Can you work these out from the drawing? Everything is in mm from the part's minimum corner. A direction names the side the tool comes from. Coordinates: 2 decimals unless noted, no trailing zeros. Loops run counter-clockwise (first coordinate to the right, second up) from the corner with the lowest first, then second, coordinate; pieces in that order, holes last.
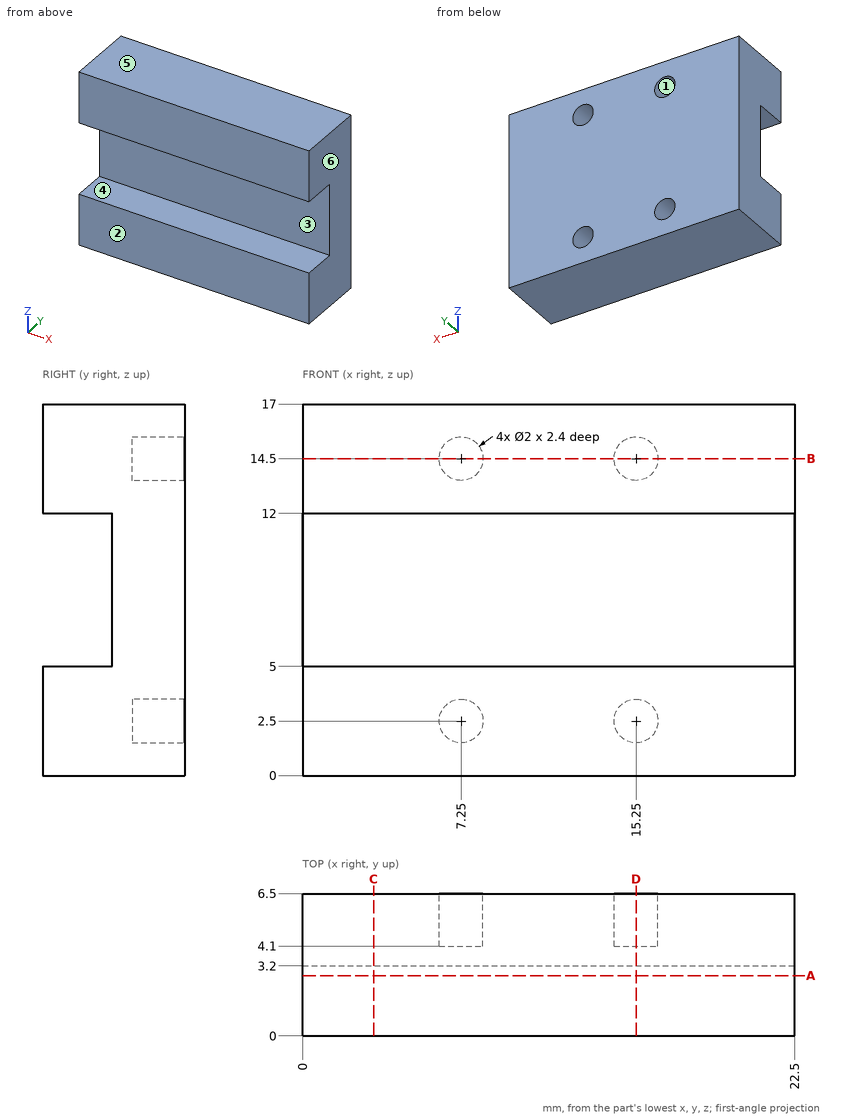
(1) Imagine slicing it at C-C, the plane x = 3.25. Write out the boundary of the cut face in (y, z).
Answers:
outline: (0, 0) - (6.5, 0) - (6.5, 17) - (0, 17) - (0, 12) - (3.2, 12) - (3.2, 5) - (0, 5) - close
(2) Imagine slicing it at D-D, the plane x = 15.25. Write out the boundary of the cut face in (y, z).
Answers:
outline: (0, 0) - (6.5, 0) - (6.5, 1.5) - (4.1, 1.5) - (4.1, 3.5) - (6.5, 3.5) - (6.5, 13.5) - (4.1, 13.5) - (4.1, 15.5) - (6.5, 15.5) - (6.5, 17) - (0, 17) - (0, 12) - (3.2, 12) - (3.2, 5) - (0, 5) - close
(3) I need wall thicknesses on probe 1 along X at (y, z) = (4.7, 14.5); probe 2 along Z at (x, y) = (15.5, 5); probe 3 along Z at (x, y) = (3, 2.25). Which ranges of each line are inside material? Lowest first, please.
Answers:
probe 1: x = 0 to 6.25, 8.25 to 14.25, 16.25 to 22.5
probe 2: z = 0 to 1.53, 3.47 to 13.53, 15.47 to 17
probe 3: z = 0 to 5, 12 to 17
(4) Imagine slicing it at A-A, the plane y = 2.75. Write out the boundary of the cut face in (x, z).
Answers:
outline: (0, 0) - (22.5, 0) - (22.5, 5) - (0, 5) - close; (0, 12) - (22.5, 12) - (22.5, 17) - (0, 17) - close
(5) Which directions (+Z, -Z, +X, -X, +Y, -Y) give clear straight access to the entire face, cutting with the end or side of a thin tool? Please do the marked faces 1 and 2.
Answers:
face 1: +Y
face 2: +Z, -Z, +X, -X, -Y
(6) Imagine slicing it at B-B, the plane z = 14.5. Write out the boundary of the cut face in (x, y).
Answers:
outline: (0, 0) - (22.5, 0) - (22.5, 6.5) - (16.25, 6.5) - (16.25, 4.1) - (14.25, 4.1) - (14.25, 6.5) - (8.25, 6.5) - (8.25, 4.1) - (6.25, 4.1) - (6.25, 6.5) - (0, 6.5) - close
(7) We'd pull the mould along Z, two halves only. Please class the marked faces 3, 4, 5 and 6: +Z half, -Z half, draft (parallel to the pull), parting line (faces both ways), or undercut.
Answers:
face 3: undercut
face 4: undercut
face 5: +Z half
face 6: draft
(8) For pin 1 (1.6 mm diameter, centred on x = 7.25, z = 2.5, fed in from +Y); pin 2 (2 mm diameter, centred on x = 16, z = 9, fed in from -Y), each with a flat end and sliding along its axis, tell me the tip position at first contact or that it passes through.
Answers:
pin 1: stops at y = 4.1
pin 2: stops at y = 3.2
